```python
from build123d import *

# Parameters (mm, degrees)
F0_R     = 12.748205
F1_DEPTH = 70
F3_DEPTH = 25
F4_R     = 5


with BuildPart() as f1:
    # F0 (on Top) → F1 (new body)
    with BuildSketch(Plane.XY):
        with BuildLine():
            ThreePointArc((-44.670311, 31.952813), (-63.008855, -10.972032), (-19.818391, 6.731877))
            ThreePointArc((-19.818391, 6.731877), (-20.780013, 13.630178), (-23.591557, 20.002501))
            ThreePointArc((-23.591557, 20.002501), (-32.601998, 28.674496), (-44.670311, 31.952813))
        make_face()
        with Locations((-45.042067, 6.731877)):
            Circle(F0_R, mode=Mode.SUBTRACT)
        with BuildLine():
            ThreePointArc((-44.670311, 31.952813), (-32.601998, 28.674496), (-23.591557, 20.002501))
            Line((-23.591557, 20.002501), (49.636481, 20.002501))
            Line((49.636481, 20.002501), (49.636481, 30.562731))
            Line((49.636481, 30.562731), (-44.670311, 31.952813))
        make_face()
    extrude(amount=F1_DEPTH)

    # F2 (on face) → F3 (cut)
    with BuildSketch(Plane.XZ.offset(-20.002501)):
        with BuildLine():
            Line((49.636481, 21.729333), (49.636481, 52.236743))
            Line((49.636481, 52.236743), (6.763435, 52.236743))
            ThreePointArc((6.763435, 52.236743), (-6.231204, 35.915426), (9.065881, 21.729333))
            Line((9.065881, 21.729333), (49.636481, 21.729333))
        make_face()
    extrude(amount=-F3_DEPTH, mode=Mode.SUBTRACT)

    # F4
    f4_edges = [f1.edges().sort_by_distance(p)[0] for p in [
        (49.636481, 25.282616, 70),
        (49.636481, 25.282616, 0),
    ]]
    fillet(f4_edges, radius=F4_R)


solid = f1.part
```
Part model, mm, in its own coordinate system. A direction names the side the tool comes from. Round coordinates to 2 decimals unless told otherwise and drop trailing zeros. Order: outer loops, then holes, each group sorted by start corner. A loop starts at its lowest first (then second) coordinate and runs counter-clockwise, first axis right, second up. Notation, with made-up numbers: M 80,-29 L 88,-29 A20 cw 88,-7 Z; hole C 42,81.25 d6. An arc over 180 degrees is marked long. Put each result on its own line as item: value. Start each with the question number.
1. Slice it at B-B on x = 32. List the corners of the cut face in (y, z), then the cut area to 3 significant figures.
2. Slice it at C-C on z = 50.5. List the corners of the cut face in (x, y).
3. Drill centre lines: probe 1 along X at (y, z) = (16.5, 11.5); probe 2 along Y at (x, z) = (-33.5, 56.5); probe 3 along X at (y, z) = (3, 40.5). Where is each one in solid material? Low to high. Write a range as [from, to].
4. Tool access for faces 3 (the face through (-4, 20.003, 27)), 4 (the face through (-26, 13, 0)), 5 (the face through (29, 26, 21.729)): list every direction of +Z, -Z, +X, -X, +Y, -Y with a clear straight run to the whole face (end or side of a thin tool).
5. Slice it at A-A on y = 5. List the corners of the cut face in (x, z).
6. Drop flat-ended pins along their axis: pin 1 (23 mm diameter, centred on x = -45.04, y = 6.73, fed in from -Z); pin 2 (1.5 mm diameter, centred on y = 23.5, z = 48, fed in from +X); pin 3 (2 mm diameter, centred on x = -45, z = 51.5, fed in from +Y); pin 4 (4 mm diameter, centred on x = -40.5, z = 22, fed in from -Y). Give the stop position or say it passes through.
7. Two-plate mould, pull along Y, no slides. Class faces 1 (the face through (-32.883, 10.561, 34.51)), 2 (the face through (29, 26, 52.237)): +Y half, -Y half, draft (parallel to the pull), parting line (faces both ways), or undercut.
8. Slice it at D-D on y = 25.5. List the corners of the cut face in (x, z), then the cut area to 3 significant figures.
Findings:
1. outline: M 20,0 L 30.82,0 L 30.82,21.73 L 20,21.73 Z; M 20,52.24 L 30.82,52.24 L 30.82,70 L 20,70 Z
1. area: 427 mm2
2. outline: M -44.67,31.95 A25.22 ccw long -19.82,6.73 A25.22 ccw -23.59,20 L 1.65,20 L 1.65,31.27 Z; hole C -45.04,6.73 d25.5
3. probe 1: [-68.3, -53.23], [-36.85, -21.79]
3. probe 2: [-15.7, 1.32], [12.14, 31.79]
3. probe 3: [-69.99, -57.23], [-32.85, -20.1]
4. face 3: +Z, -Z, +X
4. face 4: -Z, +X, -X, +Y, -Y
4. face 5: +X, +Y, -Y
5. outline: M -70.21,0 L -57.67,0 L -57.67,70 L -70.21,70 Z; M -32.41,0 L -19.88,0 L -19.88,70 L -32.41,70 Z
6. pin 1: through
6. pin 2: x = -0.88
6. pin 3: y = 31.96
6. pin 4: y = -18.36
7. face 1: undercut
7. face 2: draft
8. outline: M -61.89,0 L 44.64,0 A5 ccw 49.64,5 L 49.64,21.73 L 9.07,21.73 A15.34 cw 6.76,52.24 L 49.64,52.24 L 49.64,65 A5 ccw 44.64,70 L -61.89,70 Z
8. area: 6,190 mm2
